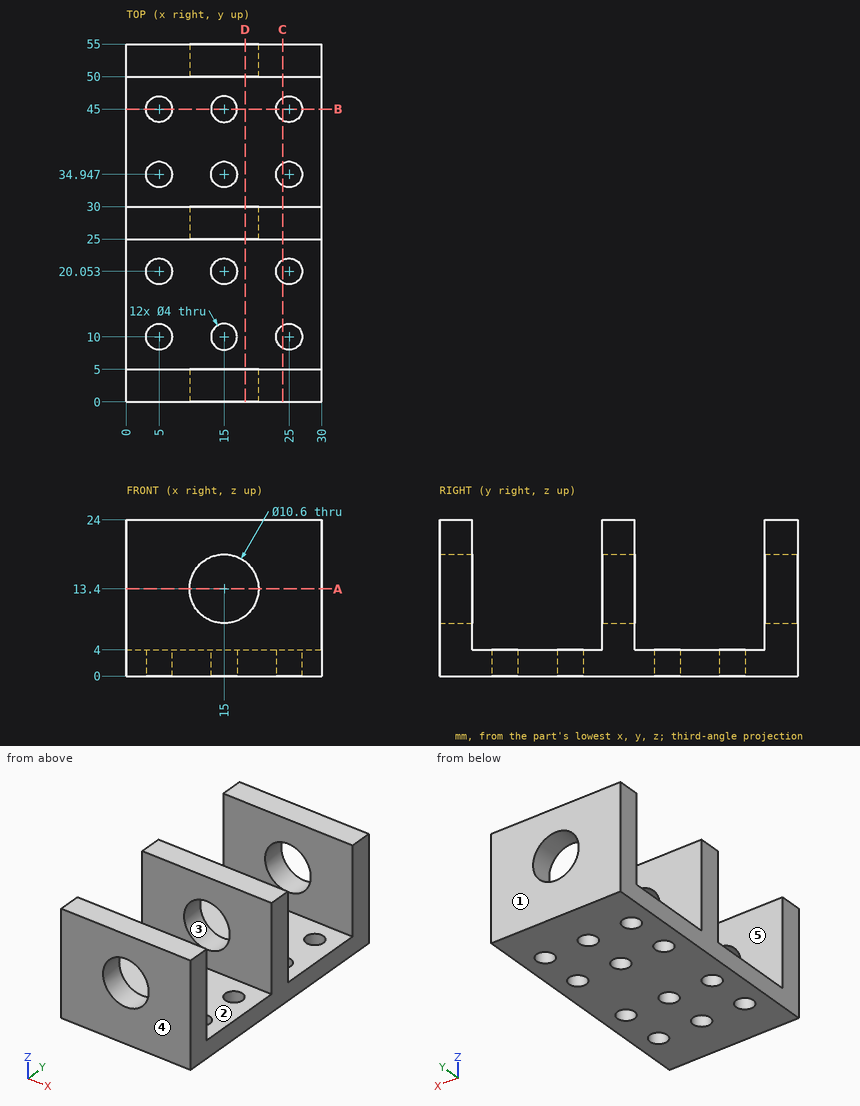
Input: dimensioned drawing with shaded views. Units: mm. Origin: part minimum x, y, z. A direction names the side the tool comes from. Round coordinates to 2 decimals unless told otherwise and drop trailing zeros. Loops run counter-clockwise (first coordinate to the right, second up) from the corner with the lowest first, then second, coordinate; pieces in that order, holes last. Notation, with made-up numbers: (14.5, 18.25) -> (62.5, 18.25) arc R21 cw to (62.5, 34.25) -> close; hole circle Ø11 at (-33.75, 57). An arc over 180 degrees is marked (long way). One line per item, written item: value.
(1) Material intervals for line 1 (Y direction, x = 25, z = 2.35); line 2 (Y direction, x = 4, z = 19.75); line 3 (Z direction, x = 2.75, y = 12), sorted ascending. Write a range as [from, to].
Geometry check:
line 1: [0, 8], [12, 18.05], [22.05, 32.95], [36.95, 43], [47, 55]
line 2: [0, 5], [25, 30], [50, 55]
line 3: [0, 4]
(2) Pin query (flat end, axial travel): pin 1 (6 mm diameter, centred on x = 15.5, y = 13.5, fed in from +Z); pin 2 (2.5 mm diameter, centred on x = 15, y = 45, fed in from +Z). Return the tip coordinate at first contact, or that it passes through.
Geometry check:
pin 1: z = 4
pin 2: through
(3) Set-up query: the marked faces 1 and 2. Return all of +Z, -Z, +X, -X, +Y, -Y with unobstructed straight access to the full face (end or side cutting, diameter ignored); none if empty.
Geometry check:
face 1: +Z, -Z, +X, -X, +Y
face 2: +Z, +X, -X
(4) Section D-D (x = 18.25). Return the cut outline in (y, z), plus the area to 3 significant figures.
Geometry check:
outline: (0, 0) -> (55, 0) -> (55, 9.21) -> (50, 9.21) -> (50, 4) -> (30, 4) -> (30, 9.21) -> (25, 9.21) -> (25, 4) -> (5, 4) -> (5, 9.21) -> (0, 9.21) -> close; (0, 17.59) -> (5, 17.59) -> (5, 24) -> (0, 24) -> close; (25, 17.59) -> (30, 17.59) -> (30, 24) -> (25, 24) -> close; (50, 17.59) -> (55, 17.59) -> (55, 24) -> (50, 24) -> close
area: 394 mm2
(5) Section C-C (x = 24). Return the cut outline in (y, z).
Geometry check:
outline: (0, 0) -> (8.27, 0) -> (8.27, 4) -> (5, 4) -> (5, 24) -> (0, 24) -> close; (11.73, 0) -> (18.32, 0) -> (18.32, 4) -> (11.73, 4) -> close; (21.79, 0) -> (33.21, 0) -> (33.21, 4) -> (30, 4) -> (30, 24) -> (25, 24) -> (25, 4) -> (21.79, 4) -> close; (36.68, 0) -> (43.27, 0) -> (43.27, 4) -> (36.68, 4) -> close; (46.73, 0) -> (55, 0) -> (55, 24) -> (50, 24) -> (50, 4) -> (46.73, 4) -> close
(6) Section A-A (z = 13.4). Return the cut outline in (x, y), plus the area to 3 significant figures.
Geometry check:
outline: (0, 0) -> (9.7, 0) -> (9.7, 5) -> (0, 5) -> close; (0, 25) -> (9.7, 25) -> (9.7, 30) -> (0, 30) -> close; (0, 50) -> (9.7, 50) -> (9.7, 55) -> (0, 55) -> close; (20.3, 0) -> (30, 0) -> (30, 5) -> (20.3, 5) -> close; (20.3, 25) -> (30, 25) -> (30, 30) -> (20.3, 30) -> close; (20.3, 50) -> (30, 50) -> (30, 55) -> (20.3, 55) -> close
area: 291 mm2
(7) Mould query, pull axis Y, two halves, no side actions, for the marked faces 3, 4 and 5. Classes: pulls with the +Y half, pulls with the -Y half, needs draft (parallel to the pull), parting line crosses it, or undercut.
Geometry check:
face 3: needs draft
face 4: pulls with the -Y half
face 5: undercut
(8) Section B-B (y = 45). Return the cut outline in (x, z), plus the area to 3 significant figures.
Geometry check:
outline: (0, 0) -> (3, 0) -> (3, 4) -> (0, 4) -> close; (7, 0) -> (13, 0) -> (13, 4) -> (7, 4) -> close; (17, 0) -> (23, 0) -> (23, 4) -> (17, 4) -> close; (27, 0) -> (30, 0) -> (30, 4) -> (27, 4) -> close
area: 72.0 mm2
